Part model, mm, in its own coordinate system. A direction names the side the tool comes from. Give positions to 0.01 mm unless a question says otherwise; leave off trailing zeros. Write each loop counter-clockwise with the first axis right and the second up, starting at its lowest first coordinate (ties: lowest second). Pieces come first, ordered by that corner, then holes. Notation, with made-up numbers: M 45,45.25 L 58,45.25 A31 cw 58,74.25 Z; hole C -22,33 d11. An arc over 180 degrees is marked long. Use a Markdown table: item, result.
```python
from build123d import *

# Parameters (mm, degrees)
F0_W     = 50.8
F0_H     = 101.6
F1_DEPTH = 19.05
F2_R     = 6.35
F3_DEPTH = 6.35
F5_DEPTH = 6.858


with BuildPart() as f1:
    # F0 (on Front) → F1 (new body)
    with BuildSketch(Plane.XZ):
        with Locations((25.4, 50.8)):
            Rectangle(F0_W, F0_H)
    extrude(amount=F1_DEPTH)

    # F2 (on face) → F3 (join)
    with BuildSketch(Plane.XZ.offset(19.05)):
        with Locations((12.7, 88.9)):
            Circle(F2_R)
        with Locations((38.1, 88.9)):
            Circle(F2_R)
        with Locations((12.7, 63.5)):
            Circle(F2_R)
        with Locations((38.1, 63.5)):
            Circle(F2_R)
        with Locations((12.7, 38.1)):
            Circle(F2_R)
        with Locations((38.1, 38.1)):
            Circle(F2_R)
        with Locations((12.7, 12.7)):
            Circle(F2_R)
        with Locations((38.1, 12.7)):
            Circle(F2_R)
    extrude(amount=F3_DEPTH)

    # F4 (on face) → F5 (cut)
    with BuildSketch(Plane(origin=(0, 0, 0), x_dir=(-1, 0, 0), z_dir=(0, 1, 0))):
        with BuildLine():
            Line((-12.7, 95.25), (-38.1, 95.25))
            ThreePointArc((-38.1, 95.25), (-42.590128, 93.390128), (-44.45, 88.9))
            Line((-44.45, 88.9), (-44.45, 12.7))
            ThreePointArc((-44.45, 12.7), (-42.590128, 8.209872), (-38.1, 6.35))
            Line((-38.1, 6.35), (-12.7, 6.35))
            ThreePointArc((-12.7, 6.35), (-8.209872, 8.209872), (-6.35, 12.7))
            Line((-6.35, 12.7), (-6.35, 88.9))
            ThreePointArc((-6.35, 88.9), (-8.209872, 93.390128), (-12.7, 95.25))
        make_face()
    extrude(amount=-F5_DEPTH, mode=Mode.SUBTRACT)


solid = f1.part
```
1. Cut at B-B, the plane x = 9. Give the cut face in (y, z).
Findings below:
| item | result |
|---|---|
| outline | M -25.4,7.54 L -19.05,7.54 L -19.05,0 L 0,0 L 0,7.54 L -6.86,7.54 L -6.86,94.06 L 0,94.06 L 0,101.6 L -19.05,101.6 L -19.05,94.06 L -25.4,94.06 L -25.4,83.74 L -19.05,83.74 L -19.05,68.66 L -25.4,68.66 L -25.4,58.34 L -19.05,58.34 L -19.05,43.26 L -25.4,43.26 L -25.4,32.94 L -19.05,32.94 L -19.05,17.86 L -25.4,17.86 Z |
2. Drill centre lines: L1, parallel to X at y = -2, z = 83; L2, parallel to Z at x = 7, y = -21; L3, parallel to Z at x = 16.5, y = -4. Where is each one in solid material? Low to high.
Findings below:
| item | result |
|---|---|
| L1 | 0 to 6.35, 44.45 to 50.8 |
| L2 | 9.9 to 15.5, 35.3 to 40.9, 60.7 to 66.3, 86.1 to 91.7 |
| L3 | 0 to 6.35, 95.25 to 101.6 |
3. Drop flat-ended pins along their axis: P1, Ø6, axis at y = -4.5, z = 91, coming from the -X side; P2, Ø19, axis at x = 22, z = 51, coming from the +Y side. Give the stop position or say it passes through.
Findings below:
| item | result |
|---|---|
| P1 | x = 0 |
| P2 | y = -6.86 |
4. Cut at C-C, the plane z = 27. Give the cut face in (x, y).
Findings below:
| item | result |
|---|---|
| outline | M 0,-19.05 L 50.8,-19.05 L 50.8,0 L 44.45,0 L 44.45,-6.86 L 6.35,-6.86 L 6.35,0 L 0,0 Z |
5. Cut at A-A, the plane z = 38.1. Give the cut face in (x, y), then the cut area to 3 significant figures.
Findings below:
| item | result |
|---|---|
| outline | M 0,-19.05 L 6.35,-19.05 L 6.35,-25.4 L 19.05,-25.4 L 19.05,-19.05 L 31.75,-19.05 L 31.75,-25.4 L 44.45,-25.4 L 44.45,-19.05 L 50.8,-19.05 L 50.8,0 L 44.45,0 L 44.45,-6.86 L 6.35,-6.86 L 6.35,0 L 0,0 Z |
| area | 868 mm2 |
6. Cut at D-D, the plane x = 40. Give the cut face in (y, z), then the cut area to 3 significant figures.
Findings below:
| item | result |
|---|---|
| outline | M -25.4,6.64 L -19.05,6.64 L -19.05,0 L 0,0 L 0,6.64 L -6.86,6.64 L -6.86,94.96 L 0,94.96 L 0,101.6 L -19.05,101.6 L -19.05,94.96 L -25.4,94.96 L -25.4,82.84 L -19.05,82.84 L -19.05,69.56 L -25.4,69.56 L -25.4,57.44 L -19.05,57.44 L -19.05,44.16 L -25.4,44.16 L -25.4,32.04 L -19.05,32.04 L -19.05,18.76 L -25.4,18.76 Z |
| area | 1,640 mm2 |
7. Two-plate mould, pull along Z, no slides. Class faces 4 (the flat face through (13, -25.4, 38)), 5 (the flat face through (25, -9, 101.6)), 6 (the flat face through (26, -3, 6.35)): released by +Z, released by -Z, zero draft, split by the parting line, or undercut.
Findings below:
| item | result |
|---|---|
| face 4 | zero draft |
| face 5 | released by +Z |
| face 6 | undercut |
8. Tool access for faces 1 (the cylindrical face through (11.32, -22.18, 57.3)), 2 (the flat face through (0, -9, 50)), 3 (the flat face through (6.35, -3, 50)): list every direction of +Z, -Z, +X, -X, +Y, -Y with a clear straight run to the whole face (end or side of a thin tool).
Findings below:
| item | result |
|---|---|
| face 1 | -Y |
| face 2 | +Z, -Z, -X, +Y, -Y |
| face 3 | +Y |
